Geometry check sheet. Reference: the model listing, model coordinates, mm. A direction names the side the tool comes from. Give positions to 0.01 mm unless a question says otherwise; leave off trailing zeros. Write each loop counter-clockwise with the first axis right and the second up, starting at its lowest first coordinate (ties: lowest second). Pieces come first, ordered by that corner, then holes. Notation, with made-up numbers: (43, -34.75) -> (74, -34.75) arc R29 ccw to (74, -2.75) -> close; hole circle Ø1 at (18.25, 13.5). An arc over 180 degrees is marked (long way). Use a Markdown table: item, result. Add a question column.
from build123d import *

# Parameters (mm, degrees)
SKETCH2_W           = 10
SKETCH2_H           = 90
BOSS_EXTRUDE1_DEPTH = 10
SKETCH3_W           = 10
SKETCH3_H           = 60
BOSS_EXTRUDE2_DEPTH = 10
BOSS_EXTRUDE3_DEPTH = 10
CUT_EXTRUDE5_START  = -8
CUT_EXTRUDE5_DEPTH  = 2
CUT_EXTRUDE6_DEPTH  = 2
SKETCH4_3_R         = 2.5
CUT_EXTRUDE1_DEPTH  = 10
CUT_EXTRUDE2_START  = -2.5
SKETCH4_5_R         = 1.5
CUT_EXTRUDE2_DEPTH  = 5
CUT_EXTRUDE3_DEPTH  = 107.338519192
FILLET3_R           = 5.25
FILLET4_R           = 5.25
SKETCH4_7_R         = 2.5
CUT_EXTRUDE4_DEPTH  = 106.904850242
FILLET5_R           = 1


# Some blends are built 0.0001 mm under size
with BuildPart() as part:
    # Sketch2 → Boss-Extrude1 (new body)
    with BuildSketch(Plane(origin=(0, 0, 0), x_dir=(1, 0, 0), z_dir=(0, 1, 0))):
        Rectangle(SKETCH2_W, SKETCH2_H)
    extrude(amount=BOSS_EXTRUDE1_DEPTH)

    # Sketch3 → Boss-Extrude2 (add)
    with BuildSketch(Plane(origin=(0, -3.907083998, 0.341825557), x_dir=(1, 0, 0), z_dir=(0, -0.9961946980917459, 0.08715574274765504))):
        with Locations((0, 74.828761414)):
            Rectangle(SKETCH3_W, SKETCH3_H)
    extrude(amount=-BOSS_EXTRUDE2_DEPTH)

    # Sketch4 → Boss-Extrude3 (add)
    with BuildSketch(Plane(origin=(5, 0, 0), x_dir=(0, 0, -1), z_dir=(1, 0, 0))):
        Polygon((-103.900124458, 15.191291546), (-44.563390571, 10), (45, 10), (-45.073853215, 14.973874535), align=None)
    extrude(amount=-BOSS_EXTRUDE3_DEPTH)

    # Sketch6 → Cut-Extrude5 (cut)
    with BuildSketch(Plane(origin=(5, 0, 0), x_dir=(0, 0, -1), z_dir=(1, 0, 0)).offset(CUT_EXTRUDE5_START)):
        Polygon((-103.900124458, 15.191291546), (-104.771681886, 5.229344565), (-84.847787924, 3.48622971), (-83.830217328, 15.117114837), align=None)
    extrude(amount=-CUT_EXTRUDE5_DEPTH, mode=Mode.SUBTRACT)

    # Sketch6<2> → Cut-Extrude6 (cut)
    with BuildSketch(Plane(origin=(5, 0, 0), x_dir=(0, 0, -1), z_dir=(1, 0, 0))):
        Polygon((-103.900124458, 15.191291546), (-104.771681886, 5.229344565), (-84.847787924, 3.48622971), (-83.830217328, 15.117114837), align=None)
    extrude(amount=-CUT_EXTRUDE6_DEPTH, mode=Mode.SUBTRACT)

    # Sketch4<3> → Cut-Extrude1 (cut)
    with BuildSketch(Plane(origin=(5, 0, 0), x_dir=(0, 0, -1), z_dir=(1, 0, 0))):
        with Locations((-97.467522719, 10)):
            Circle(SKETCH4_3_R)
    extrude(amount=-CUT_EXTRUDE1_DEPTH, mode=Mode.SUBTRACT)

    # Sketch4<5> → Cut-Extrude2 (cut)
    with BuildSketch(Plane(origin=(5, 0, 0), x_dir=(0, 0, -1), z_dir=(1, 0, 0)).offset(CUT_EXTRUDE2_START)):
        with BuildLine():
            Line((-44.537121893, 14.944236253), (-36.742124975, 6.709179338))
            ThreePointArc((-36.742124975, 6.709179338), (-34.672491645, 5.773472347), (-32.540320007, 6.556271045))
            Line((-32.540320007, 6.556271045), (-24.563390571, 13.841287616))
            Line((-24.563390571, 13.841287616), (-44.537121893, 14.944236253))
        make_face()
        with Locations((-34.563390571, 8.77148785)):
            Circle(SKETCH4_5_R, mode=Mode.SUBTRACT)
    extrude(amount=-CUT_EXTRUDE2_DEPTH, mode=Mode.SUBTRACT)

    # Sketch4<6> → Cut-Extrude3 (cut, through all)
    with BuildSketch(Plane(origin=(5, 0, 0), x_dir=(0, 0, -1), z_dir=(1, 0, 0))):
        with BuildLine():
            ThreePointArc((-33.702717638, 10), (-34.563390571, 10.27148785), (-35.424063503, 10))
            Line((-35.424063503, 10), (-33.702717638, 10))
        make_face()
        with BuildLine():
            Line((-33.702717638, 10), (-35.424063503, 10))
            ThreePointArc((-35.424063503, 10), (-35.255846563, 7.440884716), (-33.063390571, 8.77148785))
            ThreePointArc((-33.063390571, 8.77148785), (-33.232787437, 9.463943842), (-33.702717638, 10))
        make_face()
    extrude(amount=-CUT_EXTRUDE3_DEPTH, mode=Mode.SUBTRACT)

    # Fillet3
    # the kernel refuses this fillet: 5.25 mm, written as the material it takes off along each edge
    with BuildSketch(Plane(origin=(16.125, 5.229344565, 104.771681886), x_dir=(0, -0.08715574274765522, -0.9961946980917458), z_dir=(-1, 0, 0))) as fillet3_piece_1:
        with BuildLine():
            CenterArc((FILLET3_R, -FILLET3_R), FILLET3_R, 90, 90)
            Line((0, -FILLET3_R), (0, 0))
            Line((0, 0), (FILLET3_R, 0))
        make_face()
    extrude(amount=32.25, mode=Mode.SUBTRACT)
    with BuildSketch(Plane(origin=(15.07154221, 15.191291546, 103.900124458), x_dir=(0, -0.003695891671652919, -0.9999931701690523), z_dir=(-1, 0, 0))) as fillet3_piece_2:
        with BuildLine():
            CenterArc((FILLET3_R * 0.91973654932, FILLET3_R), FILLET3_R, 184.788240524, 85.211759476)
            Line((-FILLET3_R * 0.0767734631138, FILLET3_R * 0.916526680199), (0, 0))
            Line((0, 0), (FILLET3_R * 0.91973654932, 0))
        make_face()
    extrude(amount=30.14308442, mode=Mode.SUBTRACT)

    # Fillet4
    # the kernel refuses this fillet: 5.25 mm, written as the material it takes off along each edge
    with BuildSketch(Plane(origin=(-18.125, 0, -45), x_dir=(0, 1, 0), z_dir=(1, 0, 0))) as fillet4_piece_1:
        with BuildLine():
            CenterArc((FILLET4_R, FILLET4_R), FILLET4_R, 180, 90)
            Line((0, FILLET4_R), (0, 0))
            Line((0, 0), (FILLET4_R, 0))
        make_face()
    extrude(amount=36.25, mode=Mode.SUBTRACT)
    with BuildSketch(Plane(origin=(-17.420233463, 10, -45), x_dir=(0, -1, 0), z_dir=(1, 0, 0))) as fillet4_piece_2:
        with BuildLine():
            CenterArc((FILLET4_R * 0.946303501909, -FILLET4_R), FILLET4_R, 90, 86.839339304)
            Line((-FILLET4_R * 0.0521753539947, -FILLET4_R * 0.944864037923), (0, 0))
            Line((0, 0), (FILLET4_R * 0.946303501909, 0))
        make_face()
    extrude(amount=34.840466925, mode=Mode.SUBTRACT)

    # Sketch4<7> → Cut-Extrude4 (cut, through all)
    with BuildSketch(Plane(origin=(5, 0, 0), x_dir=(0, 0, -1), z_dir=(1, 0, 0))):
        with Locations((38, 5)):
            Circle(SKETCH4_7_R)
    extrude(amount=-CUT_EXTRUDE4_DEPTH, mode=Mode.SUBTRACT)

    # Fillet5
    fillet5_edges = [part.edges().sort_by_distance(p)[0] for p in [
        (-3, 9.301672273, 84.339002626),
        (-5, 9.301672273, 84.339002626),
        (3, 9.301672273, 84.339002626),
        (5, 9.301672273, 84.339002626),
    ]]
    fillet(fillet5_edges, radius=FILLET5_R - 0.0001)  # a hair under: the kernel refuses the full size


solid = part.part
1) Sectioned sample at B-B, the plane z = -38. Enter the section's corners in (x, y).
2) Draft check along X on faces 3 (the face through (-0.1, 8.6, -43.6)), 4 (the face through (2.5, 11, 35)), 5 (the face through (5, 8, 20)). Enter one of: +X half, -X half, draft (parallel to the pull), parting line (faces both ways), or undercut.
3) Gauge pin test, flat ends, axial feed: P1, Ø2, axis at x = 0.5, z = 24, coming from the +Y side; P2, Ø6, axis at y = 10, z = 97.47, coming from the -X side; P3, Ø5, axis at x = 0.5, z = 75.5, coming from the +Y side; P4, Ø4, axis at y = 5, z = -38, coming from the -X side. Record the tip position at first contact, or that the pin passes through.
4) Sectioned sample at A-A, the plane x = 0.25. Enter the section's corners in (y, z).
5) Material ranges on probe 1 along Z at (x, y) = (2.25, 8); probe 2 along Z at (x, y) = (-1.5, 6.5); probe 3 along X at (y, z) = (12.25, 94.5), recorded low to high. Write a range as [from, to].
6) Tool access check on faces 1 (the face through (0.035, 10.148, 28.608)), 2 (the face through (-0.07, 1.46, -43.383)). Record the directions out of +Z, -Z, +X, -X, +Y, -Y that give a thin tool (end or side, any length) a straight path to the whole face; none if there is none.
Check values:
| question | item | result |
|---|---|---|
| 1 | outline | (-5, 0) -> (5, 0) -> (5, 2.5) -> (-5, 2.5) -> close; (-5, 7.5) -> (5, 7.5) -> (5, 10.39) -> (-5, 10.39) -> close |
| 2 | face 3 | draft |
| 2 | face 4 | undercut |
| 2 | face 5 | +X half |
| 3 | P1 | y = 13.84 |
| 3 | P2 | x = -3 |
| 3 | P3 | y = 15.1 |
| 3 | P4 | through |
| 4 | outline | (0, -39.75) arc R5.25 ccw to (5.14, -45) arc R5.25 ccw to (10.27, -40.04) -> (13.84, 24.56) -> (6.56, 32.54) arc R3 cw to (6.71, 36.74) -> (14.94, 44.54) -> (14.97, 45.07) -> (15.17, 99.07) arc R5.25 ccw to (10.42, 104.32) arc R5.25 ccw to (4.77, 99.54) -> (0, 45) -> close; hole circle Ø5 at (5, -38); hole circle Ø5 at (10, 97.47) |
| 5 | probe 1 | [-44.08, 30.96], [37.96, 95.97], [98.97, 103.94] |
| 5 | probe 2 | [-44.79, -40], [-36, 32.6], [36.52, 103] |
| 5 | probe 3 | [-3, 3] |
| 6 | face 1 | +Y |
| 6 | face 2 | -Z, +X, -X, -Y |
